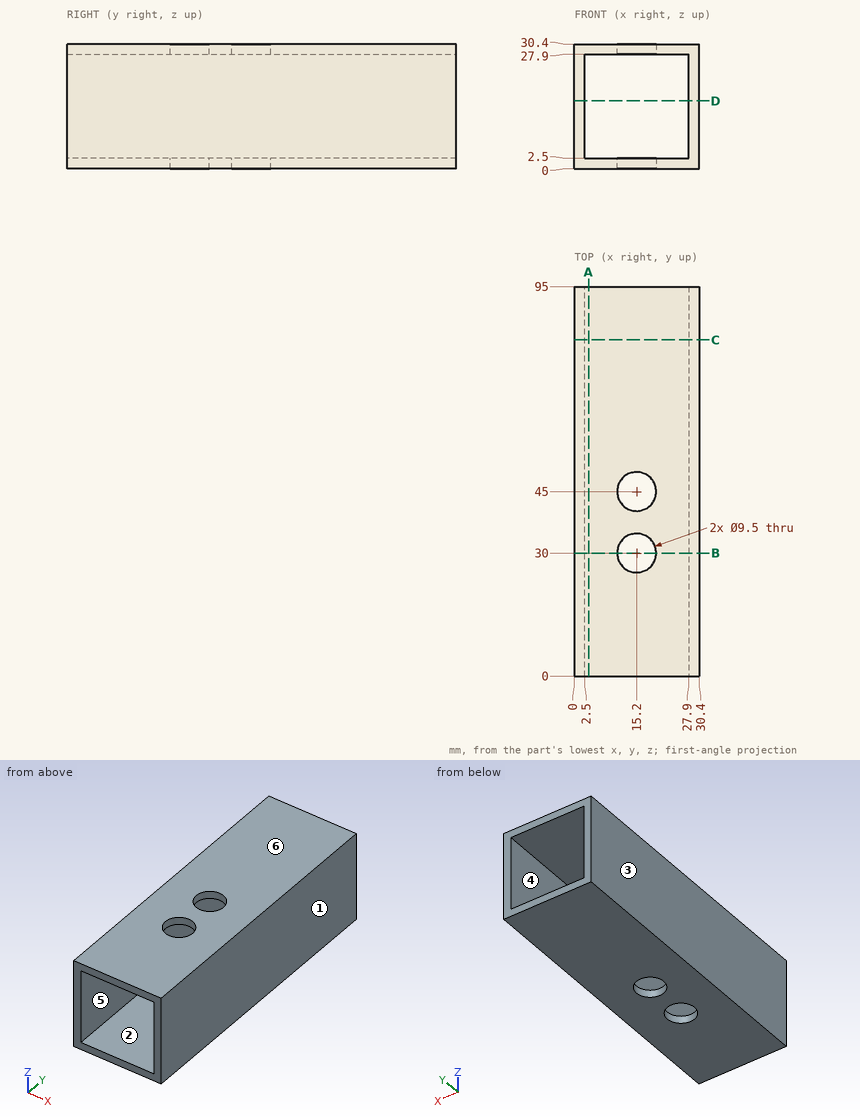
Input: dimensioned drawing with shaded views. Units: mm. Origin: part minimum x, y, z. A direction names the side the tool comes from. Round coordinates to 2 decimals unless told otherwise and drop trailing zeros. Loops run counter-clockwise (first coordinate to the right, second up) from the corner with the lowest first, then second, coordinate; pieces in that order, holes last. Notation, with made-up numbers: (11, 4) -> (17, 4) arc R5 ccw to (17, 8) -> close; hole circle Ø9 at (51, 22.25). An arc over 180 degrees is marked (long way). Answer as a JSON object with one key per item and string values. Group by question number.
Q1. Section query A-A (x = 3.5). Output: boundary loops of the cut face in (y, z).
Q2. Mould query, pull axis Z, two halves, no side actions, for the marked faces 3, 4, 5 and 6. Classes: pulls with the +Z half, pulls with the -Z half, needs draft (parallel to the pull), parting line crosses it, or undercut.
Q3. Access query for the marked faces 1 and 2. Directions: +Z, -Z, +X, -X, +Y, -Y. A direction counts if a zero-diameter tool reaches every point of the face in a straight line with its end or side. Return the directions, or none.
Q4. Section query B-B (y = 30). Output: boundary loops of the cut face in (x, z), plus the area to 4 significant figures.
Q5. Section query D-D (z = 16.5). Output: boundary loops of the cut face in (x, y).
Q6. Ray query, line 1 (Y direction, x = 15.2, z = 29.1); line 2 (X direction, y = 50.5, z = 4.5). Return the intervals inside material, ascending. Write a range as from..to.
Q7. Section query C-C (y = 82). Output: boundary loops of the cut face in (x, z), plus the area to 3 significant figures.
Completed:
{
 "1": {"outline": "(0, 0) -> (95, 0) -> (95, 2.5) -> (0, 2.5) -> close; (0, 27.9) -> (95, 27.9) -> (95, 30.4) -> (0, 30.4) -> close"},
 "2": {"face 3": "needs draft", "face 4": "undercut", "face 5": "undercut", "face 6": "pulls with the +Z half"},
 "3": {"face 1": "+Z, -Z, +X, +Y, -Y", "face 2": "+Y, -Y"},
 "4": {"outline": "(0, 0) -> (10.45, 0) -> (10.45, 2.5) -> (2.5, 2.5) -> (2.5, 27.9) -> (10.45, 27.9) -> (10.45, 30.4) -> (0, 30.4) -> close; (19.95, 0) -> (30.4, 0) -> (30.4, 30.4) -> (19.95, 30.4) -> (19.95, 27.9) -> (27.9, 27.9) -> (27.9, 2.5) -> (19.95, 2.5) -> close", "area": "231.5 mm²"},
 "5": {"outline": "(0, 0) -> (2.5, 0) -> (2.5, 95) -> (0, 95) -> close; (27.9, 0) -> (30.4, 0) -> (30.4, 95) -> (27.9, 95) -> close"},
 "6": {"line 1": "0..25.25, 34.75..40.25, 49.75..95", "line 2": "0..2.5, 27.9..30.4"},
 "7": {"outline": "(0, 0) -> (30.4, 0) -> (30.4, 30.4) -> (0, 30.4) -> close; hole (2.5, 2.5) -> (27.9, 2.5) -> (27.9, 27.9) -> (2.5, 27.9) -> close", "area": "279 mm²"}
}
